from build123d import *

# Parameters (mm, degrees)
F2_R     = 0.69999
F3_R     = 1.1
F4_DEPTH = 5.701


# Not quite as in the source:
# - a fillet or chamfer is up to 0.001 mm smaller than in the source, because OpenCascade refuses the exact size


with BuildPart() as f1:
    # F0 (on Front) → F1 (revolve)
    with BuildSketch(Plane.XZ):
        Polygon((-4.8, 0), (0, 0), (0, 5.7), (-2.5, 5.7), (-2.5, 4.9), (-5.5, 4.9), (-5.5, 4.1), (-4.8, 4.1), (-4.8, 3.4), (-3.25, 2.65), (-3.25, 1.45), (-4.8, 0.7), align=None)
    revolve(axis=Axis((0, 0, 2.85), (0, 0, -1)))

    # F2 (radius 0.7 in the source; OpenCascade refuses exactly that, so slightly less here)
    f2_edges = [f1.edges().sort_by_distance(p)[0] for p in [
        (4.8, 0, 4.1),
    ]]
    fillet(f2_edges, radius=F2_R)

    # F3 (on face) → F4 (cut, through all)
    with BuildSketch(Plane.XY.offset(5.7)):
        Circle(F3_R)
    extrude(amount=-F4_DEPTH, mode=Mode.SUBTRACT)


solid = f1.part
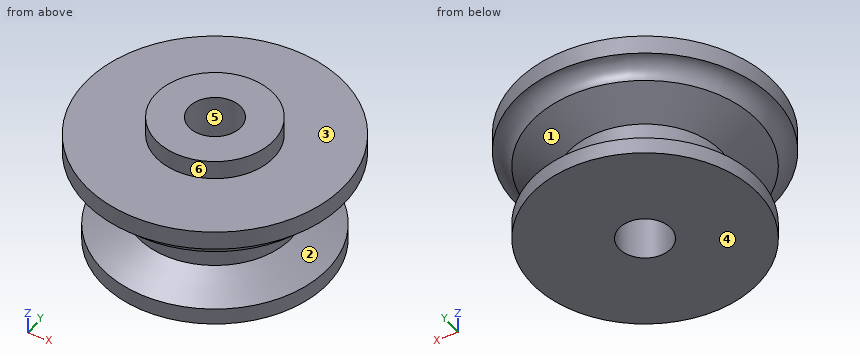
Design review of the part built by this model. Coordinates are the model's own, in mm. Face numbers are marked on the shaded views. A direction names the side the tool comes from. Round coordinates to 2 decimals unless told otherwise and drop trailing zeros. Write each loop counter-clockwise with the first axis right and the second up, starting at its lowest first coordinate (ties: lowest second). Pieces come first, ordered by that corner, then holes.
Item 1: Wall thickness on L1, parallel to Y at x = 0, z = 4.35; L2, parallel to Y at x = 0, z = 2.35; L3, parallel to Z at x = -1.5, y = -2.75: over which ranges is each line inside the solid? List them lowest first.
Item 2: Consider section D-D on z = 5.15. Give the boundary of the cut face in (x, y), and give its area (3 significant figures).
Item 3: Consider section C-C on z = 2.8. Give the boundary of the cut face in (x, y).
Item 4: Draft analysis for pull direction Z (two halves, no side actions). For the marked faces 1, 2, 3 and 4, state which applies: released by +Z, released by -Z, zero draft, split by the parting line, or undercut.
Item 5: For the marked faces 5 and 6, list the 3-axis set-ups (+Z, -Z, +X, -X, +Y, -Y) from which the entire face can be reached by the end or side of a thin tool; tool diameter is ignored.
Check values:
1. L1: y = -5.5 to -1.1, 1.1 to 5.5
1. L2: y = -3.25 to -1.1, 1.1 to 3.25
1. L3: z = 0 to 4.9
2. outline: circle Ø5 at (0, 0); hole circle Ø2.2 at (0, 0)
2. area: 15.8 mm2
3. outline: circle Ø7.12 at (0, 0); hole circle Ø2.2 at (0, 0)
4. face 1: undercut
4. face 2: undercut
4. face 3: released by +Z
4. face 4: released by -Z
5. face 5: +Z, -Z
5. face 6: +Z
